from build123d import *

# Parameters (mm, degrees)
SKETCH1_W           = 23
SKETCH1_H           = 23
BOSS_EXTRUDE1_DEPTH = 1.6
FILLET1_R           = 2
CUT_EXTRUDE1_REACH  = 18.342
SKETCH2_R           = 1.75
SKETCH3_W           = 4.3
SKETCH3_H           = 5
BOSS_EXTRUDE2_DEPTH = 1.6


with BuildPart() as part:
    # Sketch1 → Boss-Extrude1 (new body)
    with BuildSketch(Plane(origin=(0, 0, 0), x_dir=(1, 0, 0), z_dir=(0, 1, 0))):
        Rectangle(SKETCH1_W, SKETCH1_H)
    extrude(amount=BOSS_EXTRUDE1_DEPTH)

    # Fillet1
    fillet1_edges = [part.edges().sort_by_distance(p)[0] for p in [
        (11.5, 0.8, 11.5),
        (-11.5, 0.8, 11.5),
        (-11.5, 0.8, -11.5),
        (11.5, 0.8, -11.5),
    ]]
    fillet(fillet1_edges, radius=FILLET1_R)

    # Sketch2 → Cut-Extrude1 (cut, up to next)
    with BuildSketch(Plane(origin=(0, 1.6, 0), x_dir=(1, 0, 0), z_dir=(0, 1, 0)), mode=Mode.PRIVATE) as cut_extrude1_sk1:
        with Locations(Location((-8, 8.25, 0), (0, 0, 270))):
            Circle(SKETCH2_R)
    cut_extrude1_tool1 = extrude(cut_extrude1_sk1.sketch, amount=-CUT_EXTRUDE1_REACH, mode=Mode.PRIVATE) & part.part
    # Sketch2 → Cut-Extrude1 (cut, up to next)
    with BuildSketch(Plane(origin=(0, 1.6, 0), x_dir=(1, 0, 0), z_dir=(0, 1, 0)), mode=Mode.PRIVATE) as cut_extrude1_sk2:
        with Locations(Location((8, 8.25, 0), (0, 0, 270))):
            Circle(SKETCH2_R)
    cut_extrude1_tool2 = extrude(cut_extrude1_sk2.sketch, amount=-CUT_EXTRUDE1_REACH, mode=Mode.PRIVATE) & part.part
    # Sketch2 → Cut-Extrude1 (cut, up to next)
    with BuildSketch(Plane(origin=(0, 1.6, 0), x_dir=(1, 0, 0), z_dir=(0, 1, 0)), mode=Mode.PRIVATE) as cut_extrude1_sk3:
        with Locations(Location((8, -8.25, 0), (0, 0, 270))):
            Circle(SKETCH2_R)
    cut_extrude1_tool3 = extrude(cut_extrude1_sk3.sketch, amount=-CUT_EXTRUDE1_REACH, mode=Mode.PRIVATE) & part.part
    # Sketch2 → Cut-Extrude1 (cut, up to next)
    with BuildSketch(Plane(origin=(0, 1.6, 0), x_dir=(1, 0, 0), z_dir=(0, 1, 0)), mode=Mode.PRIVATE) as cut_extrude1_sk4:
        with Locations(Location((-8, -8.25, 0), (0, 0, 270))):
            Circle(SKETCH2_R)
    cut_extrude1_tool4 = extrude(cut_extrude1_sk4.sketch, amount=-CUT_EXTRUDE1_REACH, mode=Mode.PRIVATE) & part.part
    add(cut_extrude1_tool1.solids().sort_by_distance((-8, 1.6, -8.25))[0], mode=Mode.SUBTRACT)
    add(cut_extrude1_tool2.solids().sort_by_distance((8, 1.6, -8.25))[0], mode=Mode.SUBTRACT)
    add(cut_extrude1_tool3.solids().sort_by_distance((8, 1.6, 8.25))[0], mode=Mode.SUBTRACT)
    add(cut_extrude1_tool4.solids().sort_by_distance((-8, 1.6, 8.25))[0], mode=Mode.SUBTRACT)

    # Sketch3 → Boss-Extrude2 (add)
    with BuildSketch(Plane(origin=(0, 1.6, 0), x_dir=(1, 0, 0), z_dir=(0, 1, 0))):
        Rectangle(SKETCH3_W, SKETCH3_H)
    extrude(amount=BOSS_EXTRUDE2_DEPTH)


solid = part.part
Geometry: final body of the model. Coordinates: model frame, mm. A direction names the side the tool comes from. Round coordinates to 2 decimals unless told otherwise and drop trailing zeros. Order: outer loops, then holes, each group sorted by start corner. A loop starts at its lowest first (then second) coordinate and runs counter-clockwise, first axis right, second up. Notation, with made-up numbers: (48.25, 49) -> (83.25, 49) arc R7 ccw to (83.25, 62) -> close; hole circle Ø2 at (-0.5, 59). An arc over 180 degrees is marked (long way). Put each result on its own line as item: value. Start each with the question number.
Q1. Section A-A on z = -8.25. Return the cut outline in (x, y), and give its area (3 significant figures).
Q2. First-contact query: pin 1 (6 mm diameter, centred on x = -7.5, z = 2, fed in from +Y); pin 2 (3 mm diameter, centred on x = 8, z = 8.25, fed in from -Y). Flat tips, straight axial feed; report the tip coordinate or a pass-through.
Q3. Section B-B on x = -8. Return the cut outline in (y, z), and give its area (3 significant figures).
Q4. Section D-D on z = -1. Return the cut outline in (x, y).
Q5. Section C-C on y = 1. Return the cut outline in (x, z).
Q6. Reachability of faces 1 (the flat face through (-2.15, 2, 0)), 2 (the flat face through (0, 2, 2.5)), 3 (the flat face through (2.15, 2, 0)) from +Z, -Z, +X, -X, +Y, -Y: full face, straight path, thin tool, end or side. Return the list, or none.
Q7. Line query: probe 1 along X at (y, z) = (0.4, 8.25); probe 2 along Z at (x, y) = (-7, 1.2); probe 3 along X at (y, z) = (1.15, 7.5). Output: solid intervals per line, ascending.
Q8. Pull-direction query (Z, two-part tool) for faces 4 (the cylindrical face through (9.476, 0.811, -7.309)), 5 (the flat face through (11.5, 1, 0)), 6 (the flat face through (0, 1, -11.5)), 7 (the cylindrical face through (-8.67, 0.811, -6.633)); classes: +Z half, -Z half, draft (parallel to the pull), parting line (faces both ways), or undercut.
Ans:
1. outline: (-11.5, 0) -> (-9.75, 0) -> (-9.75, 1.6) -> (-11.5, 1.6) -> close; (-6.25, 0) -> (6.25, 0) -> (6.25, 1.6) -> (-6.25, 1.6) -> close; (9.75, 0) -> (11.5, 0) -> (11.5, 1.6) -> (9.75, 1.6) -> close
1. area: 25.6 mm2
2. pin 1: stops at y = 1.6
2. pin 2: passes through
3. outline: (0, -11.5) -> (1.6, -11.5) -> (1.6, -10) -> (0, -10) -> close; (0, -6.5) -> (1.6, -6.5) -> (1.6, 6.5) -> (0, 6.5) -> close; (0, 10) -> (1.6, 10) -> (1.6, 11.5) -> (0, 11.5) -> close
3. area: 25.6 mm2
4. outline: (-11.5, 0) -> (11.5, 0) -> (11.5, 1.6) -> (2.15, 1.6) -> (2.15, 3.2) -> (-2.15, 3.2) -> (-2.15, 1.6) -> (-11.5, 1.6) -> close
5. outline: (-11.5, -9.5) arc R2 ccw to (-9.5, -11.5) -> (9.5, -11.5) arc R2 ccw to (11.5, -9.5) -> (11.5, 9.5) arc R2 ccw to (9.5, 11.5) -> (-9.5, 11.5) arc R2 ccw to (-11.5, 9.5) -> close; hole circle Ø3.5 at (-8, -8.25); hole circle Ø3.5 at (-8, 8.25); hole circle Ø3.5 at (8, -8.25); hole circle Ø3.5 at (8, 8.25)
6. face 1: +Z, -Z, -X, +Y
6. face 2: +Z, +X, -X, +Y
6. face 3: +Z, -Z, +X, +Y
7. probe 1: x = -11.5 to -9.75, -6.25 to 6.25, 9.75 to 11.5
7. probe 2: z = -11.5 to -9.69, -6.81 to 6.81, 9.69 to 11.5
7. probe 3: x = -11.5 to -9.58, -6.42 to 6.42, 9.58 to 11.5
8. face 4: undercut
8. face 5: draft
8. face 6: -Z half
8. face 7: undercut
